from build123d import *

# Parameters (mm, degrees)
SKETCH1_R      = 4.7625
EXTRUDE1_DEPTH = 1.5


with BuildPart() as part:
    # Sketch1 → Extrude1 (new body)
    with BuildSketch(Plane.XY):
        with BuildLine():
            Line((-418.175, 991.35), (-468.975, 991.35))
            ThreePointArc((-468.975, 991.35), (-522.326206641, 1013.448793359), (-544.425, 1066.8))
            Line((-544.425, 1066.8), (-544.425, 1168.4))
            Line((-544.425, 1168.4), (-418.175, 1168.4))
            Line((-418.175, 1168.4), (-418.175, 991.35))
        make_face()
        with Locations((-444.2625, 1153.3)):
            Circle(SKETCH1_R, mode=Mode.SUBTRACT)
        with Locations((-495.0625, 1153.3)):
            Circle(SKETCH1_R, mode=Mode.SUBTRACT)
    extrude(amount=EXTRUDE1_DEPTH)


solid = part.part
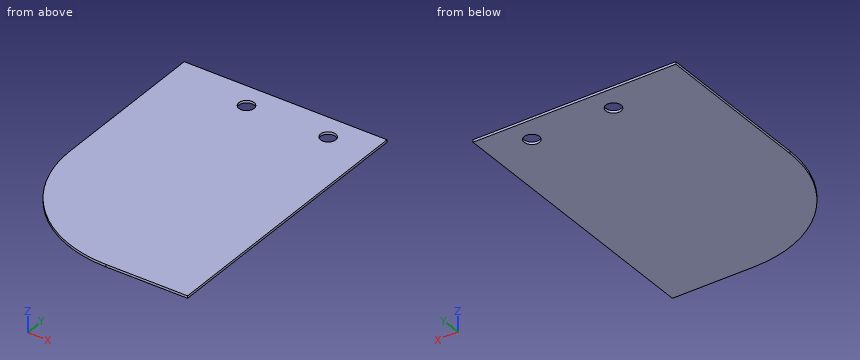
The listing builds one solid part. Answer for the finished solid, in the listing's coordinates (mm). Coordinates: 2 decimals unless noted, no trailing zeros. Loops run counter-clockwise (first coordinate to the right, second up) from the corner with the lowest first, then second, coordinate; pieces in that order, holes last. Notation, with made-up numbers: (66, 79) -> (84, 79) arc R26 ccw to (84, 118) -> close; hole circle Ø7 at (-22.5, 12.25). An arc over 180 degrees is marked (long way). Write item = value, one per line. Start each with the question number.
1) Given pin 1 Ø12.5 at (x, y) = (-495.06, 1153.3) entering from -Z, flat-ended and moving along its own axis, determine where the tip first touches the part or whether it passes through.
2) A cutting plane is placed at C-C (y = 1012.5). Give the vertices of the cut face in (x, z) (3 decimals).
3) A cutting plane is placed at B-B (z = 0.4). Count the separate pieces of the cut face and the enclosed holes in it, then the cut area to 3 significant figures.
4) Straight lines are drawn through the part: line 1 (X direction, y = 1153.3, z = 0.8) (3 decimals); line 2 (X direction, y = 1065.5, z = 0.5) (3 decimals); line 3 (Y direction, x = -446, z = 0.2). For each, find the intervals that lie inside material, in ascending order. Write a range as from..to.
5) A cutting plane is placed at A-A (y = 1153.3). Give the vertices of the cut face in (x, z) (3 decimals).
6) A cutting plane is placed at D-D (y = 1045). Give the vertices of the cut face in (x, z) (3 decimals).
Responses:
q1.pin_1 = 0
q2.outline = (-521.36, 0) -> (-418.175, 0) -> (-418.175, 1.5) -> (-521.36, 1.5) -> close
q3.separate_pieces = 1
q3.enclosed_holes = 2
q3.area = 21,000 mm²
q4.line_1 = -544.425..-499.825, -490.3..-449.025, -439.5..-418.175
q4.line_2 = -544.414..-418.175
q4.line_3 = 991.35..1148.87, 1157.73..1168.4
q5.outline = (-544.425, 0) -> (-499.825, 0) -> (-499.825, 1.5) -> (-544.425, 1.5) -> close; (-490.3, 0) -> (-449.025, 0) -> (-449.025, 1.5) -> (-490.3, 1.5) -> close; (-439.5, 0) -> (-418.175, 0) -> (-418.175, 1.5) -> (-439.5, 1.5) -> close
q6.outline = (-541.207, 0) -> (-418.175, 0) -> (-418.175, 1.5) -> (-541.207, 1.5) -> close
